```python
from build123d import *

# Parameters (mm, degrees)
F1_DEPTH = 4
F2_W     = 11
F2_H     = 151
F3_DEPTH = 4


with BuildPart() as f1:
    # F0 (on Front) → F1 (new body)
    with BuildSketch(Plane.XZ):
        Polygon((40, 4), (40, 0), (78, 0), (78, 4), (116, 4), (116, 0), (154, 0), (154, 4), (190, 4), (190, 38), (194, 38), (194, 80), (190, 80), (190, 118), (194, 118), (194, 160), (190, 160), (190, 194), (154, 194), (154, 198), (116, 198), (116, 194), (78, 194), (78, 198), (40, 198), (40, 194), (4, 194), (4, 160), (0, 160), (0, 118), (4, 118), (4, 80), (0, 80), (0, 38), (4, 38), (4, 4), align=None)
    extrude(amount=F1_DEPTH)

    # F2 (on Front) → F3 (cut)
    with BuildSketch(Plane.XZ):
        with BuildLine():
            ThreePointArc((65.992474, 171.123865), (60.492474, 176.623865), (54.992474, 171.123865))
            Line((54.992474, 171.123865), (65.992474, 171.123865))
        make_face()
        with Locations((60.492474, 95.623865)):
            Rectangle(F2_W, F2_H)
        with BuildLine():
            Line((65.992474, 20.123865), (54.992474, 20.123865))
            ThreePointArc((54.992474, 20.123865), (60.492474, 14.623865), (65.992474, 20.123865))
        make_face()
        with BuildLine():
            ThreePointArc((86.992474, 171.123865), (81.492474, 176.623865), (75.992474, 171.123865))
            Line((75.992474, 171.123865), (86.992474, 171.123865))
        make_face()
        with Locations((81.492474, 95.623865)):
            Rectangle(F2_W, F2_H)
        with BuildLine():
            Line((86.992474, 20.123865), (75.992474, 20.123865))
            ThreePointArc((75.992474, 20.123865), (81.492474, 14.623865), (86.992474, 20.123865))
        make_face()
        with BuildLine():
            ThreePointArc((107.992474, 171.123865), (102.492474, 176.623865), (96.992474, 171.123865))
            Line((96.992474, 171.123865), (107.992474, 171.123865))
        make_face()
        with Locations((102.492474, 95.623865)):
            Rectangle(F2_W, F2_H)
        with BuildLine():
            Line((107.992474, 20.123865), (96.992474, 20.123865))
            ThreePointArc((96.992474, 20.123865), (102.492474, 14.623865), (107.992474, 20.123865))
        make_face()
        with BuildLine():
            ThreePointArc((128.992474, 171.123865), (123.492474, 176.623865), (117.992474, 171.123865))
            Line((117.992474, 171.123865), (128.992474, 171.123865))
        make_face()
        with Locations((123.492474, 95.623865)):
            Rectangle(F2_W, F2_H)
        with BuildLine():
            Line((128.992474, 20.123865), (117.992474, 20.123865))
            ThreePointArc((117.992474, 20.123865), (123.492474, 14.623865), (128.992474, 20.123865))
        make_face()
        with BuildLine():
            ThreePointArc((149.992474, 171.123865), (144.492474, 176.623865), (138.992474, 171.123865))
            Line((138.992474, 171.123865), (149.992474, 171.123865))
        make_face()
        with Locations((144.492474, 95.623865)):
            Rectangle(F2_W, F2_H)
        with BuildLine():
            Line((149.992474, 20.123865), (138.992474, 20.123865))
            ThreePointArc((138.992474, 20.123865), (144.492474, 14.623865), (149.992474, 20.123865))
        make_face()
    extrude(amount=F3_DEPTH, mode=Mode.SUBTRACT)


solid = f1.part
```
Design review of the part built by this model. Coordinates are the model's own, in mm. A direction names the side the tool comes from. Give positions to 0.01 mm unless a question says otherwise; leave off trailing zeros. Order: outer loops, then holes, each group sorted by start corner. A loop starts at its lowest first (then second) coordinate and runs counter-clockwise, first axis right, second up. Notation, with made-up numbers: (31, -17.75) - (67, -17.75) arc R32 cw to (67, 10.25) - close; hole circle Ø5 at (13, -32). An arc over 180 degrees is marked (long way). Use a Markdown table: item, result. Add a question column.
(1) Machinability: for faces 1 (the face through (144.613, -1.972, 176.623)), 2 (the face through (96, 0, 100)), which of the approach directions +Z, -Z, +X, -X, +Y, -Y give a long, thin tool a straight path to every point of the face, cutting with its end or side? Answer none if there is none.
(2) Wall thickness on probe 1 along X at (y, z) = (-2.25, 171); probe 2 along X at (y, z) = (-0.3, 137); probe 3 along Z at (x, y) = (109, -0.25): over which ranges is each line inside the solid? List them lowest first. Write a range as [from, to].
(3) Add section A-A on z = 133.5. Give the boundary of the cut face in (x, y), then the cut area to 3 significant figures.
(4) Mouldability with a two-part tool opening along X and no side actions: class faces 3 (the face through (96, -4, 100)), 4 (the face through (123.372, -1.972, 14.625)) as +X half, -X half, draft (parallel to the pull), parting line (faces both ways), or undercut.
(5) Add section D-D on x = 59.5. Give the boundary of the cut face in (y, z), then the cut area to 3 significant figures.
(6) Add section C-C on y = -3. Give the number of separate pieces and of enclosed holes in the cut face, then the cut area to 3 significant figures.
(7) Add section B-B on x = 145. Give the boundary of the cut face in (y, z).
(8) Clearance check with flat-ended pins moving along their axes: P1, Ø2, axis at x = 63.5, z = 151, coming from the -Y side; P2, Ø2, axis at x = 192.5, y = -2, coming from the -Z side; P3, Ø2, axis at y = -2, z = 110, coming from the +X side; P4, Ø1.2, axis at y = -1, z = 102, coming from the -X side. State where each tip first meets the part, or that it passes through.
Report:
| question | item | result |
|---|---|---|
| 1 | face 1 | +Y, -Y |
| 1 | face 2 | +Z, -Z, +X, -X, +Y |
| 2 | probe 1 | x = [4, 54.99], [65.99, 75.99], [86.99, 96.99], [107.99, 117.99], [128.99, 138.99], [149.99, 190] |
| 2 | probe 2 | x = [0, 54.99], [65.99, 75.99], [86.99, 96.99], [107.99, 117.99], [128.99, 138.99], [149.99, 194] |
| 2 | probe 3 | z = [4, 194] |
| 3 | outline | (0, -4) - (54.99, -4) - (54.99, 0) - (0, 0) - close; (65.99, -4) - (75.99, -4) - (75.99, 0) - (65.99, 0) - close; (86.99, -4) - (96.99, -4) - (96.99, 0) - (86.99, 0) - close; (107.99, -4) - (117.99, -4) - (117.99, 0) - (107.99, 0) - close; (128.99, -4) - (138.99, -4) - (138.99, 0) - (128.99, 0) - close; (149.99, -4) - (194, -4) - (194, 0) - (149.99, 0) - close |
| 3 | area | 556 mm² |
| 4 | face 3 | draft |
| 4 | face 4 | undercut |
| 5 | outline | (-4, 0) - (0, 0) - (0, 14.71) - (-4, 14.71) - close; (-4, 176.53) - (0, 176.53) - (0, 198) - (-4, 198) - close |
| 5 | area | 145 mm² |
| 6 | separate pieces | 1 |
| 6 | enclosed holes | 5 |
| 6 | area | 27,800 mm² |
| 7 | outline | (-4, 0) - (0, 0) - (0, 14.65) - (-4, 14.65) - close; (-4, 176.6) - (0, 176.6) - (0, 198) - (-4, 198) - close |
| 8 | P1 | passes through |
| 8 | P2 | stops at z = 38 |
| 8 | P3 | stops at x = 190 |
| 8 | P4 | stops at x = 4 |
